Build history of the part. All positions in model axes, mm. Face numbers are marked on the shaded views. A direction names the side the tool comes from. Give positions to 0.01 mm unless a question says otherwise; leave off trailing zeros. Order: outer loops, then holes, each group sorted by start corner. A loop starts at its lowest first (then second) coordinate and runs counter-clockwise, first axis right, second up. Notation, with made-up numbers: (-25, -38.5) -> (14, -38.5) arc R22 ccw to (14, -13.5) -> close; hole circle Ø2 at (0, -26). An arc over 180 degrees is marked (long way). One line per item, written item: value. Start each with the question number.
(1) Probe line 1 (Z direction, x = 8818.5, y = 1276); line 2 (Y direction, x = 8644.5, z = 1547.5); line 3 (X direction, y = 1232, z = 1518). List the from-to ranges inside material, lowest first.
(2) Saw through at A-A on x = 7958.5. Give the cut face in (y, z), plus the area to 3 significant figures.
(3) Two-plate mould, pull along Y, no slides. Class the marked faces 5, 6 and 7: +Y half, -Y half, draft (parallel to the pull), parting line (faces both ways), or undercut.
(4) Pin check, flat tip, straight feed: pin 1 (12 mm diameter, centred on x = 8414, y = 1072.5, fed in from -Z). Stop position of the tip, or through.
(5) Saw through at B-B on y = 565.5. Give the cut face in (x, z).
(6) Saw through at D-D on z = 1318.5. Give the cut face in (x, y).
(7) Which spindle directions (+Z, -Z, +X, -X, +Y, -Y) get a long thin tool onto all of the face, cutting with end or side? Do the marked faces 1, 2, 3 and 4. Say none if no direction does.
(8) Saw through at C-C on x = 8719.5. Give the cut face in (y, z).
```python
from build123d import *

# Parameters (mm, degrees)
BOX3529_W        = 1200
BOX3529_H        = 900
BOX3529_DEPTH    = 500
ARRAY281_Z_COUNT = 4
ARRAY281_Z_PITCH = 550
BOX3527_W        = 400
BOX3527_H        = 600
BOX3527_DEPTH    = 2200
BOX3528_W        = 1300
BOX3528_H        = 400
BOX3528_DEPTH    = 2200


with BuildPart() as array281:
    # Box3529 → Box3529 (new body)
    with BuildSketch(Plane(origin=(8850, 1350, 0), x_dir=(-1, 0, 0), z_dir=(0, 0, 1))):
        with Locations((600, 450)):
            Rectangle(BOX3529_W, BOX3529_H)
    extrude(amount=BOX3529_DEPTH)

    # Array281 Z: Array281 ×4


with BuildPart() as array281_1:
    add(array281.part)
    with Locations(*[(0, 0, i * ARRAY281_Z_PITCH) for i in range(1, ARRAY281_Z_COUNT)]):
        add(array281.part)


with BuildPart() as box3527:
    # Box3527 → Box3527 (new body)
    with BuildSketch(Plane(origin=(8900, 1000, 0), x_dir=(-1, 0, 0), z_dir=(0, 0, 1))):
        with Locations((200, 300)):
            Rectangle(BOX3527_W, BOX3527_H)
    extrude(amount=BOX3527_DEPTH)


with BuildPart() as cut003:
    # Box3528 → Box3528 (new body)
    with BuildSketch(Plane(origin=(8900, 1400, 0), x_dir=(-1, 0, 0), z_dir=(0, 0, 1))):
        with Locations((650, 200)):
            Rectangle(BOX3528_W, BOX3528_H)
    extrude(amount=BOX3528_DEPTH)

    # Fusion015: union Box3527
    add(box3527.part)

    # Cut003: cut Array281
    add(array281_1.part, mode=Mode.SUBTRACT)


solid = cut003.part
```
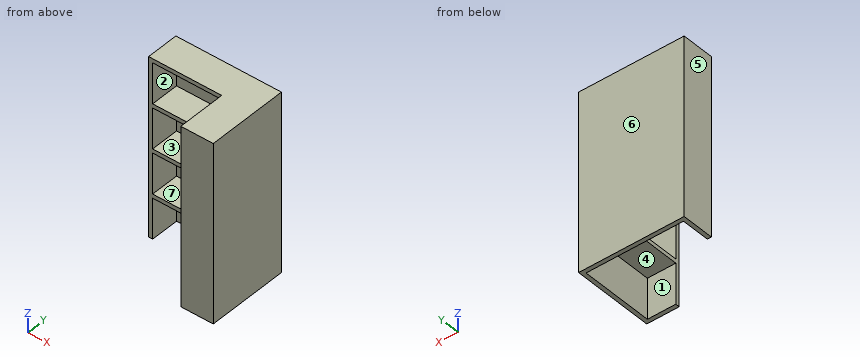
Results below:
1. line 1: z = 500 to 550, 1050 to 1100, 1600 to 1650, 2150 to 2200
1. line 2: y = 400 to 450, 1350 to 1400
1. line 3: x = 7600 to 7650, 8850 to 8900
2. outline: (1000, 500) -> (1350, 500) -> (1350, 0) -> (1400, 0) -> (1400, 2200) -> (1000, 2200) -> (1000, 2150) -> (1350, 2150) -> (1350, 1650) -> (1000, 1650) -> (1000, 1600) -> (1350, 1600) -> (1350, 1100) -> (1000, 1100) -> (1000, 1050) -> (1350, 1050) -> (1350, 550) -> (1000, 550) -> close
2. area: 180,000 mm²
3. face 5: draft
3. face 6: +Y half
3. face 7: undercut
4. pin 1: stops at z = 500
5. outline: (8500, 500) -> (8850, 500) -> (8850, 0) -> (8900, 0) -> (8900, 2200) -> (8500, 2200) -> (8500, 2150) -> (8850, 2150) -> (8850, 1650) -> (8500, 1650) -> (8500, 1600) -> (8850, 1600) -> (8850, 1100) -> (8500, 1100) -> (8500, 1050) -> (8850, 1050) -> (8850, 550) -> (8500, 550) -> close
6. outline: (7600, 1000) -> (7650, 1000) -> (7650, 1350) -> (8850, 1350) -> (8850, 450) -> (8500, 450) -> (8500, 400) -> (8900, 400) -> (8900, 1400) -> (7600, 1400) -> close
7. face 1: -Z, -X
7. face 2: -Y
7. face 3: none
7. face 4: -Z
8. outline: (400, 0) -> (450, 0) -> (450, 500) -> (1350, 500) -> (1350, 0) -> (1400, 0) -> (1400, 2200) -> (400, 2200) -> close; hole (450, 550) -> (1350, 550) -> (1350, 1050) -> (450, 1050) -> close; hole (450, 1100) -> (1350, 1100) -> (1350, 1600) -> (450, 1600) -> close; hole (450, 1650) -> (1350, 1650) -> (1350, 2150) -> (450, 2150) -> close
